Verification items for this drawing (mm, ordinates from the low corner). A direction names the side the tool comes from. Coordinates: 2 decimals unless noted, no trailing zeros. Order: outer loops, then holes, each group sorted by start corner. A loop starts at its lowest first (then second) coordinate and runs counter-clockwise, first axis right, second up. Notation, with made-up numbers: (39, -20) - (56, -20) arc R27 ccw to (56, 3) - close; hole circle Ø2 at (6.5, 36). An arc over 180 degrees is marked (long way). One line per question, with ' | ' between items. Start each with the question number.
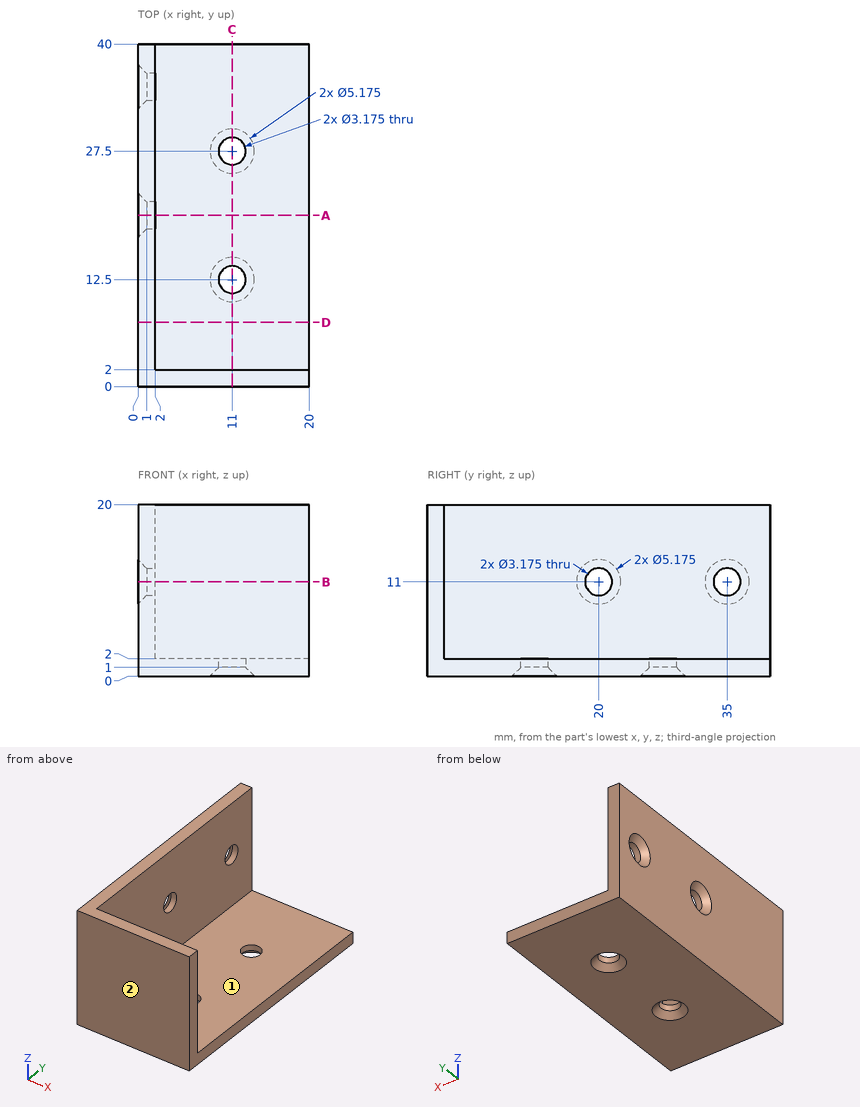
Item 1: Section check C-C (x = 11). Record the cut outline in (y, z), then the cut area to 3 significant figures.
Item 2: Section check D-D (y = 7.5). Record the cut outline in (x, z).
Item 3: Set-up check for the marked faces 1 and 2: record each of +Z, -Z, +X, -X, +Y, -Y from which the full face is reachable in a straight line by a thin tool's end or side.
Item 4: Section check B-B (z = 11). Record the cut outline in (x, y).
Item 5: Gauge pin test, flat ends, axial feed: pin 1 (1 mm diameter, centred on y = 11.5, z = 9.5, fed in from +X); pin 2 (5 mm diameter, centred on x = 9.5, y = 33.5, fed in from +Z); pin 3 (3.5 mm diameter, centred on x = 11, y = 27.5, fed in from -Z). Record the tip position at first contact, or that the pin passes through.
Item 6: Thickness scan on probe 1 along Y at (x, z) = (11, 1.5); probe 2 along Z at (x, y) = (1.75, 20); probe 3 along X at (y, z) = (29, 16). Record the ranges inside material, lowest first. Write a range as from..to.
Item 7: Section check A-A (y = 20). Record the cut outline in (x, z), then the cut area to 4 significant figures.
Completed:
1) outline: (0, 0) - (9.91, 0) - (10.91, 1) - (10.91, 2) - (2, 2) - (2, 20) - (0, 20) - close; (14.09, 1) - (15.09, 0) - (24.91, 0) - (25.91, 1) - (25.91, 2) - (14.09, 2) - close; (29.09, 1) - (30.09, 0) - (40, 0) - (40, 2) - (29.09, 2) - close | area: 101 mm^2
2) outline: (0, 0) - (20, 0) - (20, 2) - (2, 2) - (2, 20) - (0, 20) - close
3) face 1: +Z, +X, +Y | face 2: +Z, -Z, +X, -X, -Y
4) outline: (0, 0) - (20, 0) - (20, 2) - (2, 2) - (2, 18.41) - (1, 18.41) - (0, 17.41) - close; (0, 22.59) - (1, 21.59) - (2, 21.59) - (2, 33.41) - (1, 33.41) - (0, 32.41) - close; (0, 37.59) - (1, 36.59) - (2, 36.59) - (2, 40) - (0, 40) - close
5) pin 1: stops at x = 2 | pin 2: stops at z = 2 | pin 3: stops at z = 0.84
6) probe 1: y = 0..10.91, 14.09..25.91, 29.09..40 | probe 2: z = 0..9.41, 12.59..20 | probe 3: x = 0..2
7) outline: (0, 0) - (20, 0) - (20, 2) - (2, 2) - (2, 9.41) - (1, 9.41) - (0, 8.41) - close; (0, 13.59) - (1, 12.59) - (2, 12.59) - (2, 20) - (0, 20) - close | area: 68.65 mm^2
